Could you check a few things on this model? Use its own coordinates, in mm. Round coordinates to 2 decimals unless told otherwise and drop trailing zeros. Loops run counter-clockwise (first coordinate to the right, second up) from the corner with the lowest first, then second, coordinate; pieces in that order, holes last. Notation, with made-up numbers: (73, -5.75) -> (84, -5.75) arc R20 ccw to (84, 11.25) -> close; hole circle Ø3 at (47.25, 32.25). An arc over 180 degrees is marked (long way). One line per item, written item: value.
from build123d import *

# Parameters (mm, degrees)
BOSS_EXTRUDE1_DEPTH = 2


with BuildPart() as part:
    # Sketch2 → Boss-Extrude1 (new body)
    with BuildSketch(Plane(origin=(0, 0, 0), x_dir=(1, 0, 0), z_dir=(0, 1, 0))):
        with BuildLine():
            Line((33.126933041, -63.09374476), (33.126933041, -18.054684141))
            add(Edge.make_bspline(
                [(48.502275197, 18.403994452), (33.126933041, 3.028652296), (33.126933041, -18.054684141)],
                knots=[1.874843142, 1.874843142, 1.874843142, 2.666072932, 2.666072932, 2.666072932], degree=2, weights=[1, 0.922759773, 1]))
            Line((48.502275197, 18.403994452), (64.532040349, 34.433759604))
            add(Edge.make_bspline(
                [(64.532040349, 34.433759604), (90.098280745, 60), (53.804046318, 60)],
                knots=[2.359992588, 2.359992588, 2.359992588, 4.71238898, 4.71238898, 4.71238898], degree=2, weights=[1, 0.384437234, 1]))
            Line((53.804046318, 60), (-53.804046318, 60))
            add(Edge.make_bspline(
                [(-53.804046318, 60), (-90.098280745, 60), (-64.532040349, 34.433759604)],
                knots=[1.570796327, 1.570796327, 1.570796327, 3.923192719, 3.923192719, 3.923192719], degree=2, weights=[1, 0.384437234, 1]))
            Line((-64.532040349, 34.433759604), (-48.502275197, 18.403994452))
            add(Edge.make_bspline(
                [(-33.126933041, -18.054684141), (-33.126933041, 3.028652296), (-48.502275197, 18.403994452)],
                knots=[3.617112375, 3.617112375, 3.617112375, 4.408342165, 4.408342165, 4.408342165], degree=2, weights=[1, 0.922759773, 1]))
            Line((-33.126933041, -18.054684141), (-33.126933041, -63.09374476))
            add(Edge.make_bspline(
                [(-33.126933041, -63.09374476), (-33.126933041, -77.64337492), (-18.972450653, -77.64337492)],
                knots=[2.250325805, 2.250325805, 2.250325805, 3.732484786, 3.732484786, 3.732484786], degree=2, weights=[1, 0.737740241, 1]))
            Line((-18.972450653, -77.64337492), (18.972450653, -77.64337492))
            add(Edge.make_bspline(
                [(18.972450653, -77.64337492), (33.126933041, -77.64337492), (33.126933041, -63.09374476)],
                knots=[5.692293175, 5.692293175, 5.692293175, 7.174452156, 7.174452156, 7.174452156], degree=2, weights=[1, 0.737740241, 1]))
        make_face()
    extrude(amount=-BOSS_EXTRUDE1_DEPTH)


solid = part.part
(1) I'm going to push flat-ended pins straight in: pin 1 Ø0.6 at (y, z) = (-1, 35) entering from +X; pin 2 Ø1 at (y, z) = (-1, 30) entering from -X; pin 3 Ø1 at (y, z) = (-2, 2) entering from +X. Where does each tip first touch, or does it pass through?
Recorded:
pin 1: x = 33.13
pin 2: x = -33.13
pin 3: x = 35.95
(2) If I drill on L1, parallel to X at y = -0.25, z = 38; L2, parallel to X at y = -0.55, z = 3; L3, parallel to Z at x = 46, y = -1.85, over which ranges is the centre line in solid material (lowest first)?
Recorded:
L1: -33.13 to 33.13
L2: -35.46 to 35.46
L3: -60 to -15.73
(3) If we section it at A-A, the plane z = 57.5: Please give me the cut outline in (x, y).
Recorded:
outline: (-33.13, -2) -> (33.13, -2) -> (33.13, 0) -> (-33.13, 0) -> close
